from build123d import *

# Parameters (mm, degrees)
F0_W     = 70.205692
F0_H     = 65.499166
F0_R     = 14.710247
F1_DEPTH = 25.4
F2_R     = 5.08
F3_R     = 5.08
F5_D     = 6.35


with BuildPart() as f1:
    # F0 (on Top) → F1 (new body)
    with BuildSketch(Plane.XY):
        with Locations((-1.372734, -7.648109)):
            Rectangle(F0_W, F0_H)
        Circle(F0_R, mode=Mode.SUBTRACT)
    extrude(amount=F1_DEPTH)

    # F2
    f2_edges = [f1.edges().sort_by_distance(p)[0] for p in [
        (-36.47558, 25.101474, 12.7),
    ]]
    fillet(f2_edges, radius=F2_R)

    # F3
    f3_edges = [f1.edges().sort_by_distance(p)[0] for p in [
        (33.730112, 25.101474, 12.7),
        (33.730112, -40.397692, 12.7),
        (-36.47558, -40.397692, 12.7),
    ]]
    fillet(f3_edges, radius=F3_R)

    # F5 (through all)
    with Locations(Plane.YZ.offset(33.730112)):
        with Locations((-3.10241, 16.666889), (-3.10241, 8.856437), (-10.79876, 8.856437), (-10.79876, 16.666889)):
            Hole(F5_D / 2)


solid = f1.part
Source: CAD feature listing. Evaluate the final solid. Frame: model axes, mm. Round coordinates to 2 decimals unless told otherwise and drop trailing zeros. Loops run counter-clockwise (first coordinate to the right, second up) from the corner with the lowest first, then second, coordinate; pieces in that order, holes last. Notation, with made-up numbers: (71.5, 3.5) -> (108.5, 3.5) arc R12 cw to (108.5, 20.5) -> close; hole circle Ø3 at (13, -12). An arc over 180 degrees is marked (long way). Answer as a JSON object with one key per item and string values. Group by question number.
Q1. Section query C-C (y = 1.5). Output: boundary loops of the cut face in (x, z), plus the area to 3 significant figures.
Q2. Mould query, pull axis Z, two halves, no side actions, for faces 1 (the flat face through (-10, -14, 25.4)), 2 (the cylindrical face through (-24.301, -13.827, 17.621)), 3 (the cylindrical face through (32.203, 23.653, 12.878)). Classes: pulls with the +Z half, pulls with the -Z half, needs draft (parallel to the pull), parting line crosses it, or undercut.
Q3. Section query A-A (x = 0). Output: boundary loops of the cut face in (y, z), plus the area to 3 significant figures.
Q4. Contact query for a flat-ended pin moving along its axis: P1, Ø5, axis at y = -3.1, z = 8.86, coming from the -X side. Output: stop coordinate, or through.
Q5. Ray query, line 1 (Y direction, x = 25, z = 9); line 2 (Y direction, x = 29, z = 7.25); line 3 (Y direction, x = 0, z = 15.5). Return the intervals inside material, ascending. Write a range as from..to.
Q6. Section query D-D (x = 27). Output: boundary loops of the cut face in (y, z) (3 decimals).
Q7. Section query B-B (z = 2.25). Output: boundary loops of the cut face in (x, y).
Completed:
{
 "1": {"outline": "(-36.48, 0) -> (-14.63, 0) -> (-14.63, 25.4) -> (-36.48, 25.4) -> close; (14.63, 0) -> (33.73, 0) -> (33.73, 25.4) -> (14.63, 25.4) -> close", "area": "1,040 mm²"},
 "2": {"face 1": "pulls with the +Z half", "face 2": "undercut", "face 3": "needs draft"},
 "3": {"outline": "(-40.4, 0) -> (-14.71, 0) -> (-14.71, 25.4) -> (-40.4, 25.4) -> close; (14.71, 0) -> (25.1, 0) -> (25.1, 25.4) -> (14.71, 25.4) -> close", "area": "916 mm²"},
 "4": {"P1": "through"},
 "5": {"line 1": "-40.4..-13.97, -7.63..-6.27, 0.07..25.1", "line 2": "-40.39..-13.54, -8.06..-5.84, -0.36..25.09", "line 3": "-40.4..-14.71, 14.71..25.1"},
 "6": {"outline": "(-40.398, 0) -> (25.101, 0) -> (25.101, 25.4) -> (-40.398, 25.4) -> close; hole circle Ø6.35 at (-10.799, 8.856); hole circle Ø6.35 at (-10.799, 16.667); hole circle Ø6.35 at (-3.102, 8.856); hole circle Ø6.35 at (-3.102, 16.667)"},
 "7": {"outline": "(-36.48, -35.32) arc R5.08 ccw to (-31.4, -40.4) -> (28.65, -40.4) arc R5.08 ccw to (33.73, -35.32) -> (33.73, 20.02) arc R5.08 ccw to (28.65, 25.1) -> (-31.4, 25.1) arc R5.08 ccw to (-36.48, 20.02) -> close; hole circle Ø29.42 at (0, 0)"}
}
